from build123d import *

# Parameters (mm, degrees)
PAD011_DEPTH            = 24
SKETCH036_R             = 5.3
SKETCH036_R_2           = 1.7
POCKET021_DEPTH         = 0.001
POCKET021_DEPTH_BACK    = 24.001
SKETCH034_R             = 11
SKETCH034_R_2           = 5.3
SKETCH034_R_3           = 1.7
PAD012_DEPTH            = 30
SKETCH039_R             = 7.6
SKETCH039_R_2           = 5.3
SKETCH039_R_3           = 1.7
POCKET022_DEPTH         = 30.001
POCKET022_DEPTH_BACK    = 0.001
PAD018_DEPTH            = 6
SKETCH041_W             = 5.73
SKETCH041_H             = 2.5
POCKET023_DEPTH         = 8
SKETCH042_R             = 1.5
POCKET024_DEPTH         = 12.901
POCKET025_DEPTH         = 2.6
LINEARPATTERN_COUNT     = 2
LINEARPATTERN_PITCH     = 16
BODY006_PITCH_ANGLE     = 90
BODY006_PLACEMENT_ANGLE = 90


with BuildPart() as part:
    # Sketch035 → Pad011 (new body)
    with BuildSketch(Plane.YZ):
        with BuildLine():
            Line((-18.499997, 10), (18.500003, 10))
            ThreePointArc((18.500003, -10), (28.500003, 0), (18.500003, 10))
            Line((18.500003, -10), (6.499997, -10))
            Line((-18.499997, -10), (6.499997, -10))
            ThreePointArc((-28.500003, 0), (-25.571069, -7.07107), (-18.499997, -10))
            ThreePointArc((-18.499997, 10), (-25.571069, 7.07107), (-28.500003, 0))
        make_face()
    extrude(amount=PAD011_DEPTH)

    # Sketch036 → Pocket021 (cut, two sides)
    with BuildSketch(Plane.YZ) as pocket021_sk:
        Circle(SKETCH036_R)
        with Locations((-5.65, 5.65)):
            Circle(SKETCH036_R_2)
        with Locations((5.65, 5.65)):
            Circle(SKETCH036_R_2)
        with Locations((5.65, -5.65)):
            Circle(SKETCH036_R_2)
        with Locations((-5.65, -5.65)):
            Circle(SKETCH036_R_2)
    extrude(amount=-POCKET021_DEPTH, mode=Mode.SUBTRACT)
    extrude(pocket021_sk.sketch, amount=POCKET021_DEPTH_BACK, mode=Mode.SUBTRACT)

    # Sketch034 → Pad012 (join)
    with BuildSketch(Plane.YZ):
        Circle(SKETCH034_R)
        Circle(SKETCH034_R_2, mode=Mode.SUBTRACT)
        with Locations((-5.65, 5.65)):
            Circle(SKETCH034_R_3, mode=Mode.SUBTRACT)
        with Locations((5.65, 5.65)):
            Circle(SKETCH034_R_3, mode=Mode.SUBTRACT)
        with Locations((5.65, -5.65)):
            Circle(SKETCH034_R_3, mode=Mode.SUBTRACT)
        with Locations((-5.65, -5.65)):
            Circle(SKETCH034_R_3, mode=Mode.SUBTRACT)
    extrude(amount=PAD012_DEPTH)

    # Sketch039 → Pocket022 (cut, two sides)
    with BuildSketch(Plane.YZ) as pocket022_sk:
        with Locations((18.500003, 0)):
            Circle(SKETCH039_R)
        with Locations((-18.500003, 0)):
            Circle(SKETCH039_R)
        Circle(SKETCH039_R_2)
        with Locations((-5.65, 5.65)):
            Circle(SKETCH039_R_3)
        with Locations((5.65, 5.65)):
            Circle(SKETCH039_R_3)
        with Locations((5.65, -5.65)):
            Circle(SKETCH039_R_3)
        with Locations((-5.65, -5.65)):
            Circle(SKETCH039_R_3)
    extrude(amount=POCKET022_DEPTH, mode=Mode.SUBTRACT)
    extrude(pocket022_sk.sketch, amount=-POCKET022_DEPTH_BACK, mode=Mode.SUBTRACT)

    # Sketch040 → Pad018 (join)
    with BuildSketch(Plane.YZ):
        with BuildLine():
            Line((-28.500003, 0), (-28.500003, -12.9))
            Line((-28.500003, -12.9), (6.499997, -12.9))
            Line((6.499997, -12.9), (6.499997, -10))
            Line((-18.499997, -10), (6.499997, -10))
            ThreePointArc((-28.500003, 0), (-25.571069, -7.07107), (-18.499997, -10))
        make_face()
    extrude(amount=PAD018_DEPTH)

    # Sketch041 → Pocket023 (cut)
    with BuildSketch(Plane.YZ):
        with Locations((-17.735003, -10.15)):
            Rectangle(SKETCH041_W, SKETCH041_H)
        with Locations((1.264997, -10.15)):
            Rectangle(SKETCH041_W, SKETCH041_H)
    extrude(amount=POCKET023_DEPTH, mode=Mode.SUBTRACT)

    # Sketch042 → Pocket024 (cut, through all)
    with BuildSketch(Plane.XY):
        with Locations((3, -17.735003)):
            Circle(SKETCH042_R)
        with Locations((3, 1.264997)):
            Circle(SKETCH042_R)
    extrude(amount=-POCKET024_DEPTH, mode=Mode.SUBTRACT)

    # Sketch038 → Pocket025 (cut)
    with BuildSketch(Plane.YZ.offset(26.6)):
        Polygon((1.259165, 5.148252), (11.865767, 15.754854), (15.754854, 11.865767), (5.148252, 1.259165), align=None)
        Polygon((-1.259165, 5.148252), (-11.865767, 15.754854), (-15.754854, 11.865767), (-5.148252, 1.259165), align=None)
        Polygon((1.259165, -5.148252), (5.148252, -1.259165), (15.754854, -11.865767), (11.865767, -15.754854), align=None)
        Polygon((-1.259165, -5.148252), (-11.865767, -15.754854), (-15.754854, -11.865767), (-5.148252, -1.259165), align=None)
    pocket025 = extrude(amount=-POCKET025_DEPTH, mode=Mode.SUBTRACT)

    # LinearPattern: Pocket025 ×2
    with Locations(*[(-i * LINEARPATTERN_PITCH, 0, 0) for i in range(1, LINEARPATTERN_COUNT)]):
        add(pocket025, mode=Mode.SUBTRACT)


with BuildPart() as part_1:
    # Body006 pitch: moved
    add(part.part.rotate(Axis((0, 0, 0), (0, 1, 0)), BODY006_PITCH_ANGLE))


with BuildPart() as part_2:
    # Body006 placement: moved
    add(part_1.part.moved(Location((0, 0, 30))).rotate(Axis((0, 0, 30), (0, 0, 1)), BODY006_PLACEMENT_ANGLE))


solid = part_2.part
Read the model definition and answer for the solid it produces. Units are mm, in the model's axes. A direction names the side the tool comes from. Round coordinates to 2 decimals unless told otherwise and drop trailing zeros. Write each loop counter-clockwise with the first axis right and the second up, starting at its lowest first coordinate (ties: lowest second). Pieces come first, ordered by that corner, then holes.
1. The part is cut by section B-B, the plane x = -0.5. Determine the outline of the cut face in (y, z), then the cut area to 3 significant figures.
2. Straight lines are drawn through the part: L1, parallel to Y at x = -18.5, z = 19; L2, parallel to Z at x = 4, y = -4.25; L3, parallel to Y at x = 5.65, z = 1.8. For each, find the intervals that lie inside material, in ascending order.
3. Which of the six approach directions +Z, -Z, +X, -X, +Y, -Y give full straight-line access (tool end or side, diameter ignored) to faces 4 (the face through (0, -11.4, 28.4)), 5 (the face through (3.65, -7.54, 20.68)), 6 (the face through (12, 10, 18))?
4. The part is cut by section C-C, the plane x = 8. Determine the outline of the cut face in (y, z).
5. The part is cut by section A-A, the plane x = 23.5. Determine the outline of the cut face in (y, z).
6. Given pin 1 Ø2.5 at (x, y) = (5.65, -5.65) entering from +Z (3 decimals); pin 2 Ø3 at (y, z) = (-1, 4) entering from +X; pin 3 Ø12 at (x, z) = (0.5, 6.5) entering from -Y; pin 4 Ø15.5 at (x, z) = (-9.5, 22) entering from +Y, each flat-ended and moving along its own axis, determine where each tip first touches the part or whether it passes through.
7. The part is cut by section D-D, the plane z = 27. State how many separate pieces and enclosed holes the cut face has, then the cut area to 3 significant figures.
8. Determine the mould class of faces 1 (the face through (-7.27, 6.16, 12.79)), 2 (the face through (28.5, -6, 27)), 3 (the face through (-6.5, -11, 27)) for opening direction X: pulls with the +X half, pulls with the -X half, needs draft (parallel to the pull), parting line crosses it, or undercut.
Values:
1. outline: (-12.9, 24) - (-11.4, 24) - (-11.4, 25.71) - (-12.9, 25.71) - close; (-12.9, 28.29) - (-11.4, 28.29) - (-11.4, 30) - (-12.9, 30) - close; (-10.99, 0) - (-5.28, 0) - (-5.28, 25.71) - (-8.9, 25.71) - (-8.9, 22) - (-10.99, 22) - close; (-8.9, 28.29) - (-5.28, 28.29) - (-5.28, 30) - (-8.9, 30) - close; (5.28, 0) - (10.99, 0) - (10.99, 30) - (5.28, 30) - close
1. area: 322 mm2
2. L1: y = -10 to -7.6, 7.6 to 10
2. L2: z = 0 to 3.4, 6 to 19.4, 22 to 30
2. L3: y = -9.44 to -7.35, -3.95 to 3.95, 7.35 to 9.44
3. face 4: +Z, -Z
3. face 5: none
3. face 6: +Z, -Z, +X, +Y
4. outline: (-12.9, 24) - (-10, 24) - (-10, 22) - (-4.11, 22) - (-4.11, 19.4) - (-10, 19.4) - (-10, 6) - (-4.11, 6) - (-4.11, 3.4) - (-7.55, 3.4) - (-7.55, 0) - (7.55, 0) - (7.55, 3.4) - (4.11, 3.4) - (4.11, 6) - (10, 6) - (10, 19.4) - (4.11, 19.4) - (4.11, 22) - (10, 22) - (10, 30) - (-12.9, 30) - close
5. outline: (-12.9, 24) - (-8.66, 24) - (-8.66, 6) - (-5.72, 6) - (-5.72, 30) - (-12.9, 30) - close; (5.72, 6) - (8.66, 6) - (8.66, 30) - (5.72, 30) - close
6. pin 1: passes through
6. pin 2: stops at x = 10.96
6. pin 3: stops at y = -11
6. pin 4: stops at y = 10.86
7. separate pieces: 1
7. enclosed holes: 5
7. area: 642 mm2
8. face 1: undercut
8. face 2: pulls with the +X half
8. face 3: pulls with the -X half
